```python
from build123d import *

# Parameters (mm, degrees)
SKETCH1_R           = 1.375
SKETCH1_R_2         = 1.460845326
SKETCH1_R_3         = 1.480655282
BOSS_EXTRUDE1_DEPTH = 15
BOSS_EXTRUDE2_START = -8
SKETCH2_R           = 14
SKETCH2_R_2         = 10
BOSS_EXTRUDE2_DEPTH = 8
CUT_EXTRUDE1_START  = -3
SKETCH3_R           = 14
SKETCH3_R_2         = 10
CUT_EXTRUDE1_DEPTH  = 3
SKETCH5_R           = 1.480655282
SKETCH5_R_2         = 1.375
SKETCH5_R_3         = 1.460845326
BOSS_EXTRUDE3_DEPTH = 0.5
SKETCH6_W           = 32.415484222
SKETCH6_H           = 34.71462202
CUT_EXTRUDE2_DEPTH  = 7
SKETCH7_W           = 33.435139342
SKETCH7_H           = 35.82697306
CUT_EXTRUDE3_DEPTH  = 2
BOSS_EXTRUDE4_DEPTH = 6.5
SKETCH9_R           = 3.5
SKETCH9_R_2         = 1.625
CUT_EXTRUDE4_DEPTH  = 3
SKETCH10_R          = 3
CUT_EXTRUDE5_DEPTH  = 28
SKETCH11_R          = 14.05
CUT_EXTRUDE6_DEPTH  = 3.5


with BuildPart() as part:
    # Sketch1 → Boss-Extrude1 (new body)
    with BuildSketch(Plane(origin=(0, 0, 0), x_dir=(1, 0, 0), z_dir=(0, 1, 0))):
        with BuildLine():
            Line((-15, -16.85), (15, -16.85))
            Line((15, -16.85), (15, 16.85))
            Line((15, 16.85), (-15, 16.85))
            Line((-15, 16.85), (-15, 2.633913438))
            ThreePointArc((-15, 2.633913438), (0.072875656, 13.937359865), (12.75, 0))
            ThreePointArc((12.75, 0), (0.072875656, -13.937359865), (-15, -2.633913438))
            Line((-15, -2.633913438), (-15, -16.85))
        make_face()
        with Locations(Location((-11.75, -13.5, 0), (0, 0, 270))):
            Circle(SKETCH1_R, mode=Mode.SUBTRACT)
        with Locations(Location((9.25, -13.5, 0), (0, 0, 270))):
            Circle(SKETCH1_R_2, mode=Mode.SUBTRACT)
        with Locations(Location((-11.75, 13.5, 0), (0, 0, 270))):
            Circle(SKETCH1_R, mode=Mode.SUBTRACT)
        with Locations(Location((9.25, 13.5, 0), (0, 0, 270))):
            Circle(SKETCH1_R_3, mode=Mode.SUBTRACT)
    extrude(amount=BOSS_EXTRUDE1_DEPTH)

    # Sketch2 → Boss-Extrude2 (add)
    with BuildSketch(Plane(origin=(0, 15, 0), x_dir=(1, 0, 0), z_dir=(0, 1, 0)).offset(BOSS_EXTRUDE2_START)):
        with Locations((-1.25, 0)):
            Circle(SKETCH2_R)
        with Locations(Location((-1.25, 0, 0), (0, 0, 270))):
            Circle(SKETCH2_R_2, mode=Mode.SUBTRACT)
    extrude(amount=BOSS_EXTRUDE2_DEPTH)

    # Sketch3 → Cut-Extrude1 (cut)
    with BuildSketch(Plane(origin=(0, 15, 0), x_dir=(1, 0, 0), z_dir=(0, 1, 0)).offset(CUT_EXTRUDE1_START)):
        with Locations((-1.25, 0)):
            Circle(SKETCH3_R)
        with Locations(Location((-1.25, 0, 0), (0, 0, 270))):
            Circle(SKETCH3_R_2, mode=Mode.SUBTRACT)
    extrude(amount=CUT_EXTRUDE1_DEPTH, mode=Mode.SUBTRACT)

    # Sketch5 → Boss-Extrude3 (add)
    with BuildSketch(Plane(origin=(0, 15, 0), x_dir=(1, 0, 0), z_dir=(0, 1, 0))):
        with BuildLine():
            Line((-15, 16.85), (-15, 2.633913438))
            ThreePointArc((-15, 2.633913438), (12.75, 0), (-15, -2.633913438))
            Line((-15, -2.633913438), (-15, -16.85))
            Line((-15, -16.85), (15, -16.85))
            Line((15, -16.85), (15, 16.85))
            Line((15, 16.85), (-15, 16.85))
        make_face()
        with Locations(Location((9.25, 13.5, 0), (0, 0, 270))):
            Circle(SKETCH5_R, mode=Mode.SUBTRACT)
        with Locations(Location((-11.75, -13.5, 0), (0, 0, 270))):
            Circle(SKETCH5_R_2, mode=Mode.SUBTRACT)
        with Locations(Location((-11.75, 13.5, 0), (0, 0, 270))):
            Circle(SKETCH5_R_2, mode=Mode.SUBTRACT)
        with Locations(Location((9.25, -13.5, 0), (0, 0, 270))):
            Circle(SKETCH5_R_3, mode=Mode.SUBTRACT)
    extrude(amount=BOSS_EXTRUDE3_DEPTH)

    # Sketch6 → Cut-Extrude2 (cut)
    with BuildSketch(Plane.XZ):
        Rectangle(SKETCH6_W, SKETCH6_H)
    extrude(amount=-CUT_EXTRUDE2_DEPTH, mode=Mode.SUBTRACT)

    # Sketch7 → Cut-Extrude3 (cut)
    with BuildSketch(Plane.XZ.offset(-7)):
        Rectangle(SKETCH7_W, SKETCH7_H)
    extrude(amount=-CUT_EXTRUDE3_DEPTH, mode=Mode.SUBTRACT)

    # Sketch8 → Boss-Extrude4 (add)
    with BuildSketch(Plane.XZ.offset(-9)):
        with BuildLine():
            Line((3.5, 16.85), (3.5, 20.35))
            ThreePointArc((3.5, 20.35), (2.474873725, 17.875126257), (-2.6e-08, 16.85))
            Line((-2.6e-08, 16.85), (3.5, 16.85))
        make_face()
        with BuildLine():
            ThreePointArc((-2.6e-08, 16.85), (-2.474873743, 17.875126275), (-3.5, 20.35))
            Line((-3.5, 20.35), (-3.5, 16.85))
            Line((-3.5, 16.85), (-2.6e-08, 16.85))
        make_face()
        with BuildLine():
            ThreePointArc((-1.625, 20.35), (0, 21.975), (1.625, 20.35))
            Line((1.625, 20.35), (3.5, 20.35))
            ThreePointArc((3.5, 20.35), (0, 23.85), (-3.5, 20.35))
            Line((-3.5, 20.35), (-1.625, 20.35))
        make_face()
        with BuildLine():
            Line((3.5, 20.35), (1.625, 20.35))
            ThreePointArc((1.625, 20.35), (0, 18.725), (-1.625, 20.35))
            Line((-1.625, 20.35), (-3.5, 20.35))
            ThreePointArc((-3.5, 20.35), (-2.474873743, 17.875126275), (-2.6e-08, 16.85))
            ThreePointArc((-2.6e-08, 16.85), (2.474873725, 17.875126257), (3.5, 20.35))
        make_face()
        with BuildLine():
            Line((3.5, -20.35), (3.5, -16.85))
            Line((3.5, -16.85), (0, -16.85))
            ThreePointArc((0, -16.85), (2.474873734, -17.875126266), (3.5, -20.35))
        make_face()
        with BuildLine():
            ThreePointArc((-3.5, -20.35), (-2.474873734, -17.875126266), (0, -16.85))
            Line((0, -16.85), (-3.5, -16.85))
            Line((-3.5, -16.85), (-3.5, -20.35))
        make_face()
        with BuildLine():
            ThreePointArc((-3.5, -20.35), (0, -23.85), (3.5, -20.35))
            Line((3.5, -20.35), (1.625, -20.35))
            ThreePointArc((1.625, -20.35), (0, -21.975), (-1.625, -20.35))
            Line((-1.625, -20.35), (-3.5, -20.35))
        make_face()
        with BuildLine():
            Line((1.625, -20.35), (3.5, -20.35))
            ThreePointArc((3.5, -20.35), (2.474873734, -17.875126266), (0, -16.85))
            ThreePointArc((0, -16.85), (-2.474873734, -17.875126266), (-3.5, -20.35))
            Line((-3.5, -20.35), (-1.625, -20.35))
            ThreePointArc((-1.625, -20.35), (0, -18.725), (1.625, -20.35))
        make_face()
    extrude(amount=-BOSS_EXTRUDE4_DEPTH)

    # Sketch9 → Cut-Extrude4 (cut)
    # profile 1 of 2: a face of its own
    with BuildSketch(Plane.XZ.offset(-9)):
        with Locations((0, 20.35)):
            Circle(SKETCH9_R)
        with Locations(Location((0, 20.35, 0), (0, 0, 270))):
            Circle(SKETCH9_R_2, mode=Mode.SUBTRACT)
    # profile 2 of 2: a face of its own
    with BuildSketch(Plane.XZ.offset(-9)):
        with Locations((0, -20.35)):
            Circle(SKETCH9_R)
        with Locations(Location((0, -20.35, 0), (0, 0, 270))):
            Circle(SKETCH9_R_2, mode=Mode.SUBTRACT)
    extrude(amount=-CUT_EXTRUDE4_DEPTH, mode=Mode.SUBTRACT)

    # Sketch10 → Cut-Extrude5 (cut)
    with BuildSketch(Plane.XZ.offset(-9)):
        with Locations(Location((-11.75, 13.5, 0), (0, 0, 270))):
            Circle(SKETCH10_R)
        with Locations(Location((9.25, 13.5, 0), (0, 0, 270))):
            Circle(SKETCH10_R)
        with Locations(Location((9.25, -13.5, 0), (0, 0, 270))):
            Circle(SKETCH10_R)
        with Locations(Location((-11.75, -13.5, 0), (0, 0, 270))):
            Circle(SKETCH10_R)
    extrude(amount=-CUT_EXTRUDE5_DEPTH, mode=Mode.SUBTRACT)

    # Sketch11 → Cut-Extrude6 (cut)
    with BuildSketch(Plane(origin=(0, 15.5, 0), x_dir=(1, 0, 0), z_dir=(0, 1, 0))):
        with Locations((-1.25, 0)):
            Circle(SKETCH11_R)
    extrude(amount=-CUT_EXTRUDE6_DEPTH, mode=Mode.SUBTRACT)


solid = part.part
```
Design review of the part built by this model. Coordinates are the model's own, in mm. A direction names the side the tool comes from. Round coordinates to 2 decimals unless told otherwise and drop trailing zeros. Order: outer loops, then holes, each group sorted by start corner. A loop starts at its lowest first (then second) coordinate and runs counter-clockwise, first axis right, second up. Notation, with made-up numbers: (31, 88.25) - (66, 88.25) arc R25 cw to (66, 119.25) - close; hole circle Ø9 at (-0.75, 20). An arc over 180 degrees is marked (long way). Return JSON: item names as keys, results as strings.
Q1. Consider section B-B on y = 10. Write out the cut boundary in (x, z).
Computed values:
{"outline": "(-15, -16.85) - (-3.5, -16.85) - (-3.5, -20.35) arc R3.5 cw to (3.5, -20.35) - (3.5, -16.85) - (15, -16.85) - (15, 16.85) - (3.5, 16.85) - (3.5, 20.35) arc R3.5 cw to (-3.5, 20.35) - (-3.5, 16.85) - (-15, 16.85) - (-15, 2.63) arc R14 ccw to (-15, -2.63) - close; hole circle Ø6 at (-11.75, -13.5); hole circle Ø6 at (-11.75, 13.5); hole circle Ø20 at (-1.25, 0); hole circle Ø6 at (9.25, -13.5); hole circle Ø6 at (9.25, 13.5)"}
Q2. The part is to be moulded in two halves that separate along X. For faces 6 (the cylindrical face through (-11.618, 12.204, -10.503)), 7 (the flat face through (-15, 12, 10)), 8 (the flat face through (13, 15.5, 0)), say which applies: pulls with the +X half, pulls with the -X half, needs draft (parallel to the pull), parting line crosses it, or undercut.
Computed values:
{"face 6": "undercut", "face 7": "pulls with the -X half", "face 8": "needs draft"}
Q3. Wall thickness on L1, parallel to X at y = 11.75, z = 13.5; L2, parallel to Z at x = -12, y = 11.5; L3, parallel to Z at x = -9, y = 14.25: over which ranges is each line inside the solid? List them lowest first. Write a range as [from, to].
Computed values:
{"L1": "x = [-15, -14.75], [-8.75, 6.25], [12.25, 15]", "L2": "z = [-16.85, -16.49], [-10.51, 10.51], [16.49, 16.85]", "L3": "z = [-16.85, -14.7], [-12.3, -11.72], [11.72, 12.3], [14.7, 16.85]"}
Q4. Consider section C-C on x = 9.25. Write out the cut boundary in (y, z).
Computed values:
{"outline": "(9, -16.85) - (15.5, -16.85) - (15.5, -16.5) - (9, -16.5) - close; (9, -10.5) - (15.5, -10.5) - (15.5, -9.34) - (12, -9.34) - (12, 9.34) - (15.5, 9.34) - (15.5, 10.5) - (9, 10.5) - close; (9, 16.5) - (15.5, 16.5) - (15.5, 16.85) - (9, 16.85) - close"}
Q5. Consider section A-A on z = 0. Write out the cut boundary in (x, y).
Computed values:
{"outline": "(-15.25, 9) - (-11.25, 9) - (-11.25, 12) - (-15.25, 12) - close; (8.75, 9) - (15, 9) - (15, 15.5) - (12.8, 15.5) - (12.8, 12) - (8.75, 12) - close"}
Q6. For pin 1 Ø3.5 at (x, z) = (0, 20.35) entering from -Y; pin 2 Ø10 at (x, z) = (-6.5, 5) entering from -Y; pin 3 Ø2 at (x, y) = (12, 13) entering from -Z; pin 4 Ø2 at (x, y) = (-8.5, 13) entering from +Z, all flat-tipped, find the tip position at first contact; note any pin that passes through.
Computed values:
{"pin 1": "stops at y = 12", "pin 2": "stops at y = 9", "pin 3": "stops at z = -16.85", "pin 4": "stops at z = 16.85"}
Q7. Machinability: for faces 1 (the flat face through (-3.5, 12, -19)), 2 (the flat face through (2, 12, 20)), 3 (the flat face through (-9, 12, 16.85)), 4 (the flat face through (-11, 12, -3)), 5 (the cylindrical face through (0.08, 10.48, -16.85)), which of the approach directions +Z, -Z, +X, -X, +Y, -Y give a long, thin tool a straight path to every point of the face, cutting with its end or side? Answer none if there is none.
Computed values:
{"face 1": "-Z, -X, +Y, -Y", "face 2": "+Z, -Y", "face 3": "+Z, -X, +Y, -Y", "face 4": "+Y", "face 5": "-Z, -Y"}
Q8. Consider section D-D on z = 13.5. Write out the cut boundary in (x, y), plus the area to 3 significant figures.
Computed values:
{"outline": "(-15, 9) - (-14.75, 9) - (-14.75, 15.5) - (-15, 15.5) - close; (-8.75, 9) - (6.25, 9) - (6.25, 15.5) - (2.64, 15.5) - (2.64, 12) - (-5.14, 12) - (-5.14, 15.5) - (-8.75, 15.5) - close; (12.25, 9) - (15, 9) - (15, 15.5) - (12.25, 15.5) - close", "area": "89.8 mm2"}
